Could you check a few things on this model? Use its own coordinates, in mm. Face numbers are marked on the shaded views. A direction names the side the tool comes from. Coordinates: 2 decimals unless noted, no trailing zeros. Order: outer loops, then holes, each group sorted by start corner. A loop starts at its lowest first (then second) coordinate and runs counter-clockwise, first axis right, second up. Notation, with made-up numbers: M 84.25,54 L 100.25,54 A18 ccw 100.25,89 Z; hole C 16.25,44 d7. An arc over 180 degrees is marked long. Write item = value, one per line. Start each with the question number.
from build123d import *

# Parameters (mm, degrees)
SKETCH_1_W          = 212
SKETCH_1_H          = 230
EXTRUDE_1_DEPTH     = 100
SKETCH_2_W          = 202
SKETCH_2_H          = 90
CUT_EXTRUDE_1_DEPTH = 225
SKETCH_5_R          = 2.2
CUT_EXTRUDE_4_DEPTH = 238
SKETCH_6_R          = 2.1
CUT_EXTRUDE_5_DEPTH = 237


with BuildPart() as part:
    # 草圖1 → 填料-伸長1 (new body)
    with BuildSketch(Plane.XY):
        Rectangle(SKETCH_1_W, SKETCH_1_H)
    extrude(amount=EXTRUDE_1_DEPTH)

    # 草圖2 → 除料-伸長1 (cut)
    with BuildSketch(Plane.XZ.offset(115)):
        with Locations((0, 50)):
            Rectangle(SKETCH_2_W, SKETCH_2_H)
    extrude(amount=-CUT_EXTRUDE_1_DEPTH, mode=Mode.SUBTRACT)

    # 草圖5 → 除料-伸長4 (cut)
    with BuildSketch(Plane(origin=(106, 0, 0), x_dir=(0, 0, -1), z_dir=(1, 0, 0))):
        with Locations((-69.988851691, 52.009212606)):
            Circle(SKETCH_5_R)
    extrude(amount=-CUT_EXTRUDE_4_DEPTH, mode=Mode.SUBTRACT)

    # 草圖6 → 除料-伸長5 (cut)
    with BuildSketch(Plane(origin=(106, 0, 0), x_dir=(0, 0, -1), z_dir=(1, 0, 0))):
        with Locations((-69.988851691, -32.4)):
            Circle(SKETCH_6_R)
    extrude(amount=-CUT_EXTRUDE_5_DEPTH, mode=Mode.SUBTRACT)


solid = part.part
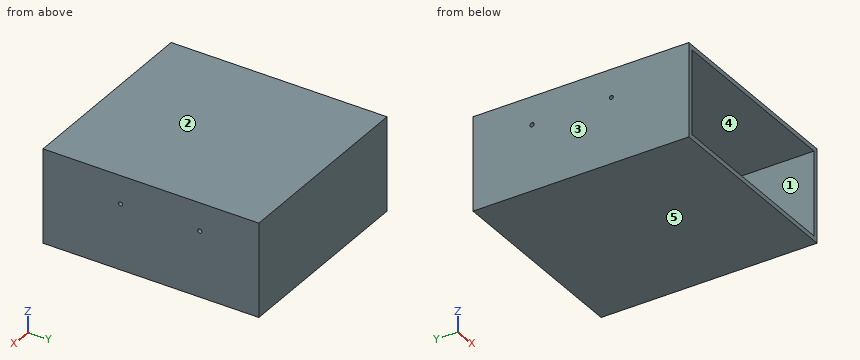
(1) Please list where these lines run through material, in increasing order: probe 1 along Z at (x, y) = (-3.5, -35); probe 2 along X at (y, z) = (61.5, 36.5); probe 3 along Y at (x, z) = (-32, 7.5). Write a range as from..to.
(2) Imagine slicing it at B-B on z = 9. List the corners of the cut face in (x, y) for me, plus the area to 3 significant figures.
(3) Imagine slicing it at C-C on x = -76. List the corners of the cut face in (y, z) for me, plus the area to 3 significant figures.
(4) Thinking about a two-plate mould opening in Z: for the marked faces 1, 2 and 3, which applies, released by +Z, released by -Z, zero draft, split by the parting line, or undercut?
(5) Imagine slicing it at A-A on y = 84. List the corners of the cut face in (x, z) for me.
(6) For the marked faces 4 and 5, which set-ups out of +Z, -Z, +X, -X, +Y, -Y let a thin tool reach every point of the face, with its end or its side?
(7) Will these pins go through, and if not, where does the flat tip stop? P1, Ø12, axis at x = 44, z = 55, coming from the -Y side; P2, Ø2.5, axis at y = 52.01, z = 69.99, coming from the +X side.
Response:
q1.probe_1 = 0..5, 95..100
q1.probe_2 = -106..-101, 101..106
q1.probe_3 = 110..115
q2.outline = M -106,-115 L -101,-115 L -101,110 L 101,110 L 101,-115 L 106,-115 L 106,115 L -106,115 Z
q2.area = 3,310 mm2
q3.outline = M -115,0 L 115,0 L 115,100 L -115,100 L -115,95 L 110,95 L 110,5 L -115,5 Z
q3.area = 2,750 mm2
q4.face_1 = undercut
q4.face_2 = released by +Z
q4.face_3 = zero draft
q5.outline = M -106,0 L 106,0 L 106,100 L -106,100 Z; hole M -101,5 L 101,5 L 101,95 L -101,95 Z
q6.face_4 = -Y
q6.face_5 = -Z, +X, -X, +Y, -Y
q7.P1 = 110
q7.P2 = through
